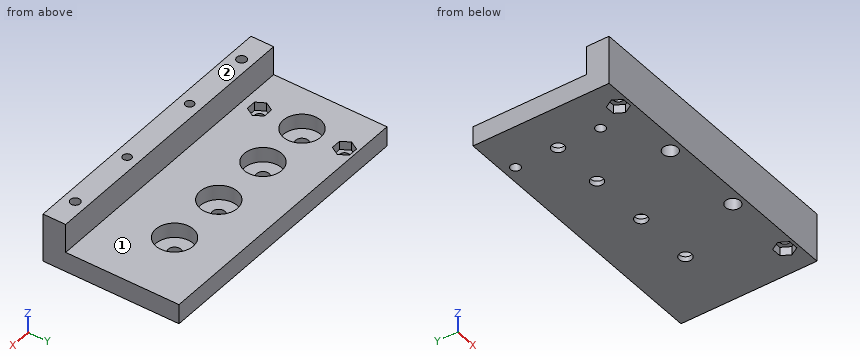
from build123d import *

# Parameters (mm, degrees)
SKETCH1_W           = 100
SKETCH1_H           = 48
BOSS_EXTRUDE1_DEPTH = 7
CUT_EXTRUDE1_REACH  = 113.144
SKETCH2_R           = 2.2
SKETCH3_W           = 100
SKETCH3_H           = 8
BOSS_EXTRUDE2_DEPTH = 10.2
SKETCH4_R           = 6.6
CUT_EXTRUDE2_DEPTH  = 5.25
SKETCH5_R           = 2.6
CUT_EXTRUDE3_DEPTH  = 7
SKETCH7_R           = 1.5
CUT_EXTRUDE4_DEPTH  = 112.391382072
CUT_EXTRUDE5_REACH  = 114.249
SKETCH8_R           = 1.7
CUT_EXTRUDE6_DEPTH  = 3
CUT_EXTRUDE7_REACH  = 114.249
SKETCH10_R          = 1.7
CUT_EXTRUDE8_DEPTH  = 3


with BuildPart() as part:
    # Sketch1 → Boss-Extrude1 (new body)
    with BuildSketch(Plane.XY):
        with Locations((50, 24)):
            Rectangle(SKETCH1_W, SKETCH1_H)
    extrude(amount=BOSS_EXTRUDE1_DEPTH)

    # Sketch2 → Cut-Extrude1 (cut, up to next)
    with BuildSketch(Plane.XY.offset(7), mode=Mode.PRIVATE) as cut_extrude1_sk1:
        with Locations((15, 29)):
            Circle(SKETCH2_R)
    cut_extrude1_tool1 = extrude(cut_extrude1_sk1.sketch, amount=-CUT_EXTRUDE1_REACH, mode=Mode.PRIVATE) & part.part
    # Sketch2 → Cut-Extrude1 (cut, up to next)
    with BuildSketch(Plane.XY.offset(7), mode=Mode.PRIVATE) as cut_extrude1_sk2:
        with Locations((33.75, 29)):
            Circle(SKETCH2_R)
    cut_extrude1_tool2 = extrude(cut_extrude1_sk2.sketch, amount=-CUT_EXTRUDE1_REACH, mode=Mode.PRIVATE) & part.part
    # Sketch2 → Cut-Extrude1 (cut, up to next)
    with BuildSketch(Plane.XY.offset(7), mode=Mode.PRIVATE) as cut_extrude1_sk3:
        with Locations((55, 29)):
            Circle(SKETCH2_R)
    cut_extrude1_tool3 = extrude(cut_extrude1_sk3.sketch, amount=-CUT_EXTRUDE1_REACH, mode=Mode.PRIVATE) & part.part
    # Sketch2 → Cut-Extrude1 (cut, up to next)
    with BuildSketch(Plane.XY.offset(7), mode=Mode.PRIVATE) as cut_extrude1_sk4:
        with Locations((76.25, 29)):
            Circle(SKETCH2_R)
    cut_extrude1_tool4 = extrude(cut_extrude1_sk4.sketch, amount=-CUT_EXTRUDE1_REACH, mode=Mode.PRIVATE) & part.part
    add(cut_extrude1_tool1.solids().sort_by_distance((15, 29, 7))[0], mode=Mode.SUBTRACT)
    add(cut_extrude1_tool2.solids().sort_by_distance((33.75, 29, 7))[0], mode=Mode.SUBTRACT)
    add(cut_extrude1_tool3.solids().sort_by_distance((55, 29, 7))[0], mode=Mode.SUBTRACT)
    add(cut_extrude1_tool4.solids().sort_by_distance((76.25, 29, 7))[0], mode=Mode.SUBTRACT)

    # Sketch3 → Boss-Extrude2 (add)
    with BuildSketch(Plane(origin=(0, 0, 0), x_dir=(-1, 0, 0), z_dir=(0, 0, -1))):
        with Locations((-50, 4)):
            Rectangle(SKETCH3_W, SKETCH3_H)
    extrude(amount=BOSS_EXTRUDE2_DEPTH)

    # Sketch4 → Cut-Extrude2 (cut)
    with BuildSketch(Plane(origin=(0, 0, 0), x_dir=(-1, 0, 0), z_dir=(0, 0, -1))):
        with Locations((-76.25, 29)):
            Circle(SKETCH4_R)
        with Locations((-55, 29)):
            Circle(SKETCH4_R)
        with Locations((-33.75, 29)):
            Circle(SKETCH4_R)
        with Locations((-15, 29)):
            Circle(SKETCH4_R)
    extrude(amount=-CUT_EXTRUDE2_DEPTH, mode=Mode.SUBTRACT)

    # Sketch5 → Cut-Extrude3 (cut)
    with BuildSketch(Plane.XY.offset(7)):
        with Locations((35.000022648, 4.052132501)):
            Circle(SKETCH5_R)
        with Locations((64.999977352, 4)):
            Circle(SKETCH5_R)
    extrude(amount=-CUT_EXTRUDE3_DEPTH, mode=Mode.SUBTRACT)

    # Sketch7 → Cut-Extrude4 (cut, through all)
    with BuildSketch(Plane.XY):
        with Locations((35.000022648, 4.052132501)):
            Circle(SKETCH7_R)
        with Locations((64.999977352, 4)):
            Circle(SKETCH7_R)
    extrude(amount=-CUT_EXTRUDE4_DEPTH, mode=Mode.SUBTRACT)

    # Sketch8 → Cut-Extrude5 (cut, up to next)
    with BuildSketch(Plane.XY.offset(7), mode=Mode.PRIVATE) as cut_extrude5_sk1:
        with Locations((10, 4.052132501)):
            Circle(SKETCH8_R)
    cut_extrude5_tool1 = extrude(cut_extrude5_sk1.sketch, amount=-CUT_EXTRUDE5_REACH, mode=Mode.PRIVATE) & part.part
    # Sketch8 → Cut-Extrude5 (cut, up to next)
    with BuildSketch(Plane.XY.offset(7), mode=Mode.PRIVATE) as cut_extrude5_sk2:
        with Locations((90, 4.052132501)):
            Circle(SKETCH8_R)
    cut_extrude5_tool2 = extrude(cut_extrude5_sk2.sketch, amount=-CUT_EXTRUDE5_REACH, mode=Mode.PRIVATE) & part.part
    add(cut_extrude5_tool1.solids().sort_by_distance((10, 4.052133, 7))[0], mode=Mode.SUBTRACT)
    add(cut_extrude5_tool2.solids().sort_by_distance((90, 4.052133, 7))[0], mode=Mode.SUBTRACT)


with BuildPart() as body_2:
    # Mirror1: mirrored copy
    add(part.part.mirror(Plane.XY.offset(-10.2)))

    # Sketch9 → Cut-Extrude6 (cut)
    with BuildSketch(Plane(origin=(0, 0, -27.4), x_dir=(-1, 0, 0), z_dir=(0, 0, -1))):
        Polygon((-88.267949192, 1.052132501), (-86.535898385, 4.052132501), (-88.267949192, 7.052132501), (-91.732050808, 7.052132501), (-93.464101615, 4.052132501), (-91.732050808, 1.052132501), align=None)
        Polygon((-13.464101615, 4.052132501), (-11.732050808, 1.052132501), (-8.267949192, 1.052132501), (-6.535898385, 4.052132501), (-8.267949192, 7.052132501), (-11.732050808, 7.052132501), align=None)
    extrude(amount=-CUT_EXTRUDE6_DEPTH, mode=Mode.SUBTRACT)

    # Sketch10 → Cut-Extrude7 (cut, up to next)
    with BuildSketch(Plane(origin=(0, 0, -27.4), x_dir=(-1, 0, 0), z_dir=(0, 0, -1)), mode=Mode.PRIVATE) as cut_extrude7_sk1:
        with Locations((-15, 44)):
            Circle(SKETCH10_R)
    cut_extrude7_tool1 = extrude(cut_extrude7_sk1.sketch, amount=-CUT_EXTRUDE7_REACH, mode=Mode.PRIVATE) & body_2.part
    # Sketch10 → Cut-Extrude7 (cut, up to next)
    with BuildSketch(Plane(origin=(0, 0, -27.4), x_dir=(-1, 0, 0), z_dir=(0, 0, -1)), mode=Mode.PRIVATE) as cut_extrude7_sk2:
        with Locations((-15, 14)):
            Circle(SKETCH10_R)
    cut_extrude7_tool2 = extrude(cut_extrude7_sk2.sketch, amount=-CUT_EXTRUDE7_REACH, mode=Mode.PRIVATE) & body_2.part
    add(cut_extrude7_tool1.solids().sort_by_distance((15, 44, -27.4))[0], mode=Mode.SUBTRACT)
    add(cut_extrude7_tool2.solids().sort_by_distance((15, 14, -27.4))[0], mode=Mode.SUBTRACT)

    # Sketch11 → Cut-Extrude8 (cut)
    with BuildSketch(Plane.XY.offset(-20.4)):
        Polygon((18.464101615, 44), (16.732050808, 47), (13.267949192, 47), (11.535898385, 44), (13.267949192, 41), (16.732050808, 41), align=None)
        Polygon((18.464101615, 14), (16.732050808, 17), (13.267949192, 17), (11.535898385, 14), (13.267949192, 11), (16.732050808, 11), align=None)
    extrude(amount=-CUT_EXTRUDE8_DEPTH, mode=Mode.SUBTRACT)


solid = body_2.part
Design review of the part built by this model. Coordinates are the model's own, in mm. Face numbers are marked on the shaded views. A direction names the side the tool comes from. Coordinates: 2 decimals unless noted, no trailing zeros. Loops run counter-clockwise (first coordinate to the right, second up) from the corner with the lowest first, then second, coordinate; pieces in that order, holes last.
Item 1: Add section B-B (x = 76.25). Write out the cut boundary in (y, z), and give its area (3 significant figures).
Completed:
outline: (0, -27.4) - (26.8, -27.4) - (26.8, -25.65) - (22.4, -25.65) - (22.4, -20.4) - (8, -20.4) - (8, -10.2) - (0, -10.2) - close; (31.2, -27.4) - (48, -27.4) - (48, -20.4) - (35.6, -20.4) - (35.6, -25.65) - (31.2, -25.65) - close
area: 341 mm2
Item 2: Add section C-C (x = 46.5). Write out the cut boundary in (y, z).
Completed:
outline: (0, -27.4) - (48, -27.4) - (48, -20.4) - (8, -20.4) - (8, -10.2) - (0, -10.2) - close
Item 3: Clearance check with flat-ended pins moving along their axes: pin 1 (6.5 mm diameter, centred on x = 35, y = 27.5, fed in from +Z); pin 2 (4 mm diameter, centred on x = 10, y = 4.05, fed in from -Z); pin 3 (1.8 mm diameter, centred on x = 14.5, y = 13, fed in from +Z). State where each tip first meets the part, or that it passes through.
Completed:
pin 1: stops at z = -25.65
pin 2: stops at z = -24.4
pin 3: stops at z = -23.4
Item 4: Add section D-D (y = 33). Write out the cut boundary in (x, z).
Completed:
outline: (0, -27.4) - (100, -27.4) - (100, -20.4) - (81.5, -20.4) - (81.5, -25.65) - (71, -25.65) - (71, -20.4) - (60.25, -20.4) - (60.25, -25.65) - (49.75, -25.65) - (49.75, -20.4) - (39, -20.4) - (39, -25.65) - (28.5, -25.65) - (28.5, -20.4) - (20.25, -20.4) - (20.25, -25.65) - (9.75, -25.65) - (9.75, -20.4) - (0, -20.4) - close
Item 5: For the marked faces 1 and 2, list the 3-axis set-ups (+Z, -Z, +X, -X, +Y, -Y) from which the entire face can be reached by the end or side of a thin tool; tool diameter is ignored.
Completed:
face 1: +Z, +X, -X, +Y
face 2: +Z, +X, -X, +Y, -Y
Item 6: Add section A-A (z = -16). Write out the cut boundary in (x, y), and give its area (3 significant figures).
Completed:
outline: (0, 0) - (100, 0) - (100, 8) - (0, 8) - close; hole circle Ø3.4 at (10, 4.05); hole circle Ø3 at (35, 4.05); hole circle Ø3 at (65, 4); hole circle Ø3.4 at (90, 4.05)
area: 768 mm2
Item 7: Wall thickness on L1, parallel to Y at x = 15, z = -26.25; L2, parallel to X at y = 44, z = -21.5; L3, parallel to Y at x = 33.75, z = -26.5: over which ranges is each line inside the solid? List them lowest first.
Completed:
L1: y = 0 to 12.3, 15.7 to 26.8, 31.2 to 42.3, 45.7 to 48
L2: x = 0 to 11.54, 18.46 to 100
L3: y = 0 to 1.77, 6.33 to 26.8, 31.2 to 48
